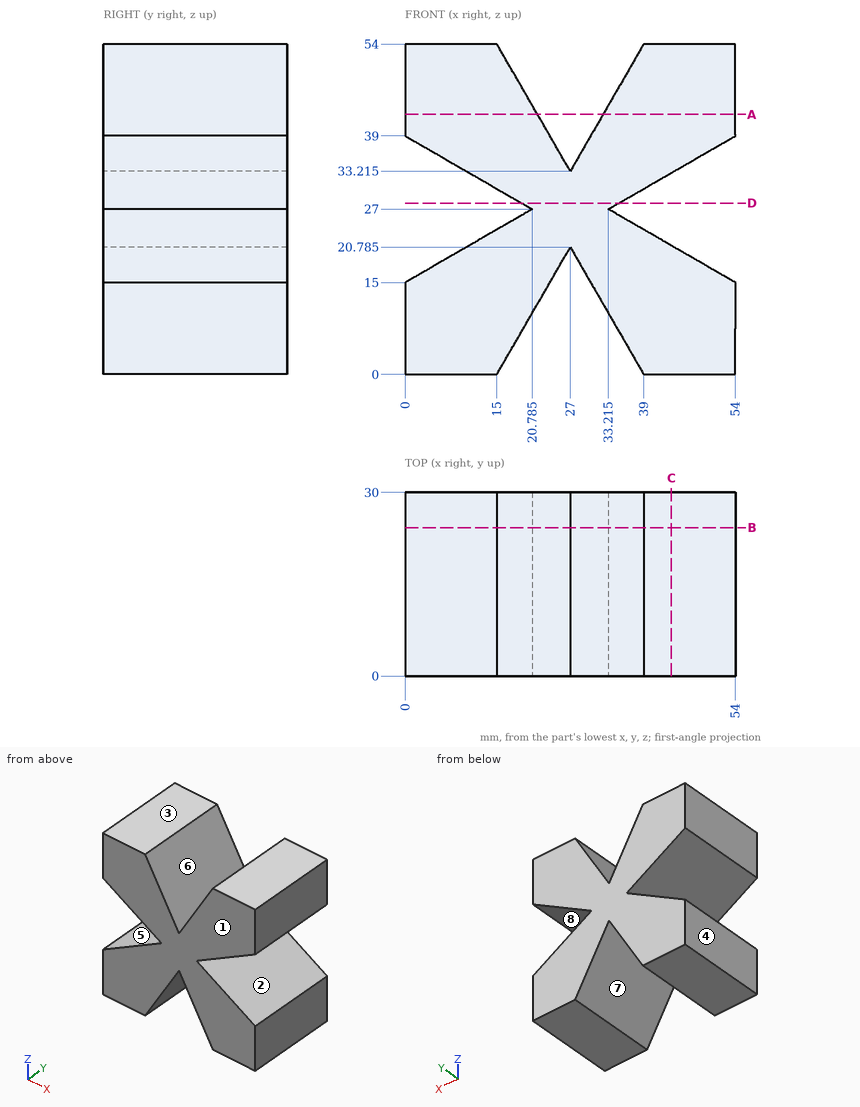
Source: three-view drawing plus pictorial views. Frame: mm from the lowest corner of the part. A direction names the side the tool comes from. Round coordinates to 2 decimals unless told otherwise and drop trailing zeros. Order: outer loops, then holes, each group sorted by start corner. A loop starts at its lowest first (then second) coordinate and runs counter-clockwise, first axis right, second up. Notation, with made-up numbers: (10, -27) - (20, -27) arc R8 cw to (20, -18) - close; hole circle Ø11 at (10, -37). An arc over 180 degrees is marked (long way). Use a Markdown table: item, result.
1. Access query for the marked faces 4, 5, 6, 7 and 8. Directions: +Z, -Z, +X, -X, +Y, -Y. A direction counts if a zero-diameter tool reaches every point of the face in a straight line with its end or side. Return the directions, or none.
Evaluation:
| item | result |
|---|---|
| face 4 | +Z, -Z, -X, +Y, -Y |
| face 5 | -X, +Y, -Y |
| face 6 | +Z, +Y, -Y |
| face 7 | -Z, +Y, -Y |
| face 8 | +X, +Y, -Y |
2. Section A-A on z = 42.5. Return the cut outline in (x, y), then the cut area to 3 significant figures.
Evaluation:
| item | result |
|---|---|
| outline | (0, 0) - (21.64, 0) - (21.64, 30) - (0, 30) - close; (32.36, 0) - (54, 0) - (54, 30) - (32.36, 30) - close |
| area | 1,300 mm^2 |
3. Mould query, pull axis Z, two halves, no side actions, for the marked faces 1, 2 and 3. Classes: +Z half, -Z half, draft (parallel to the pull), parting line (faces both ways), or undercut.
Evaluation:
| item | result |
|---|---|
| face 1 | draft |
| face 2 | undercut |
| face 3 | +Z half |
4. Section D-D on z = 28. Return the cut outline in (x, y), then the cut area to 3 significant figures.
Evaluation:
| item | result |
|---|---|
| outline | (19.05, 0) - (34.95, 0) - (34.95, 30) - (19.05, 30) - close |
| area | 477 mm^2 |
5. First-contact query: pin 1 (10 mm diameter, centred on y = 7.5, z = 30.5, fed in from +X); pin 2 (1 mm diameter, centred on y = 24.5, z = 28, fed in from +X) (1 decimal); pin 3 (1.5 mm diameter, centred on y = 13, z = 27, fed in from -X) (1 decimal); pin 4 (3 mm diameter, centred on x = 24.5, z = 44.5, fed in from +Y). Flat tips, straight axial feed; report the tip coordinate or a pass-through.
Evaluation:
| item | result |
|---|---|
| pin 1 | x = 47.94 |
| pin 2 | x = 35.8 |
| pin 3 | x = 19.5 |
| pin 4 | through |
6. Material intervals for probe 1 along X at (y, z) = (9.75, 47); probe 2 along Z at (x, y) = (35, 14.5) (1 decimal); probe 3 along X at (y, z) = (21.75, 17) (1 decimal), sorted ascending.
Evaluation:
| item | result |
|---|---|
| probe 1 | 0 to 19.04, 34.96 to 54 |
| probe 2 | 6.9 to 26, 28 to 47.1 |
| probe 3 | 3.5 to 24.8, 29.2 to 50.5 |
7. Section C-C on x = 43.5. Return the cut outline in (y, z), then the cut area to 3 significant figures.
Evaluation:
| item | result |
|---|---|
| outline | (0, 0) - (30, 0) - (30, 21.06) - (0, 21.06) - close; (0, 32.94) - (30, 32.94) - (30, 54) - (0, 54) - close |
| area | 1,260 mm^2 |
8. Section B-B on y = 24.25. Return the cut outline in (x, z) (1 decimal), then the cut area to 3 significant figures.
Evaluation:
| item | result |
|---|---|
| outline | (0, 0) - (15, 0) - (27, 20.8) - (39, 0) - (54, 0) - (54, 15) - (33.2, 27) - (54, 39) - (54, 54) - (39, 54) - (27, 33.2) - (15, 54) - (0, 54) - (0, 39) - (20.8, 27) - (0, 15) - close |
| area | 1,920 mm^2 |
